Here's how the part is built. I have some questions about the finished solid (model axes, mm). Coordinates: 2 decimals unless noted, no trailing zeros.
from build123d import *

# Parameters (mm, degrees)
F0_W     = 97.8876724839
F0_H     = 45.6908610649
F1_DEPTH = 5


with BuildPart() as f1:
    # F0 (on Top) → F1 (new body)
    with BuildSketch(Plane.XY):
        with Locations((1.2231161818, -8.5958049167)):
            Rectangle(F0_W, F0_H)
        with BuildLine():
            Line((-26.666582018, -10.6564535441), (-26.666582018, -7.637935464))
            Line((-26.666582018, -7.637935464), (-19.8852024899, -7.637935464))
            Line((-19.8852024899, -7.637935464), (-19.8852024899, -16.4989879196))
            add(Edge.make_bspline(
                [(-19.8852024899, -16.4989879196), (-21.53472724, -17.0376082461), (-22.9897502054, -17.2545525443)],
                knots=[0, 0, 0, 1, 1, 1], degree=2))
            add(Edge.make_bspline(
                [(-22.9897502054, -17.2545525443), (-24.4447731709, -17.4714968425), (-25.9633832583, -17.4714968425)],
                knots=[0, 0, 0, 1, 1, 1], degree=2))
            add(Edge.make_bspline(
                [(-25.9633832583, -17.4714968425), (-29.8309764364, -17.4714968425), (-31.8713749652, -15.1973221304)],
                knots=[0, 0, 0, 1, 1, 1], degree=2))
            add(Edge.make_bspline(
                [(-31.8713749652, -15.1973221304), (-33.9117734939, -12.9231474183), (-33.9117734939, -8.666550671)],
                knots=[0, 0, 0, 1, 1, 1], degree=2))
            add(Edge.make_bspline(
                [(-33.9117734939, -8.666550671), (-33.9117734939, -4.5296473295), (-31.5440883084, -2.2161982186)],
                knots=[0, 0, 0, 1, 1, 1], degree=2))
            add(Edge.make_bspline(
                [(-31.5440883084, -2.2161982186), (-29.1764031229, 0.0972508923), (-24.9833934975, 0.0972508923)],
                knots=[0, 0, 0, 1, 1, 1], degree=2))
            add(Edge.make_bspline(
                [(-24.9833934975, 0.0972508923), (-22.3501385677, 0.0972508923), (-19.9076450035, -0.9538068283)],
                knots=[0, 0, 0, 1, 1, 1], degree=2))
            Line((-19.9076450035, -0.9538068283), (-21.1120599004, -3.8526315024))
            add(Edge.make_bspline(
                [(-21.1120599004, -3.8526315024), (-22.9822693676, -2.9175267688), (-25.0058360111, -2.9175267688)],
                knots=[0, 0, 0, 1, 1, 1], degree=2))
            add(Edge.make_bspline(
                [(-25.0058360111, -2.9175267688), (-27.3548191019, -2.9175267688), (-28.7686974591, -4.4959835591)],
                knots=[0, 0, 0, 1, 1, 1], degree=2))
            add(Edge.make_bspline(
                [(-28.7686974591, -4.4959835591), (-30.1825758163, -6.0744403494), (-30.1825758163, -8.7376186307)],
                knots=[0, 0, 0, 1, 1, 1], degree=2))
            add(Edge.make_bspline(
                [(-30.1825758163, -8.7376186307), (-30.1825758163, -11.5204903179), (-29.0436182508, -12.9867345402)],
                knots=[0, 0, 0, 1, 1, 1], degree=2))
            add(Edge.make_bspline(
                [(-29.0436182508, -12.9867345402), (-27.9046606852, -14.4529787625), (-25.7314772844, -14.4529787625)],
                knots=[0, 0, 0, 1, 1, 1], degree=2))
            add(Edge.make_bspline(
                [(-25.7314772844, -14.4529787625), (-24.5943899283, -14.4529787625), (-23.4273792208, -14.2210727885)],
                knots=[0, 0, 0, 1, 1, 1], degree=2))
            Line((-23.4273792208, -14.2210727885), (-23.4273792208, -10.6564535441))
            Line((-23.4273792208, -10.6564535441), (-26.666582018, -10.6564535441))
        make_face(mode=Mode.SUBTRACT)
        with BuildLine():
            add(Edge.make_bspline(
                [(-11.0559435953, -4.5951046609), (-10.0217177599, -3.9236994622), (-8.8060816063, -3.9236994622)],
                knots=[0, 0, 0, 1, 1, 1], degree=2))
            add(Edge.make_bspline(
                [(-8.8060816063, -3.9236994622), (-8.080440333, -3.9236994622), (-7.6016667094, -4.0284311923)],
                knots=[0, 0, 0, 1, 1, 1], degree=2))
            Line((-7.6016667094, -4.0284311923), (-7.8709768727, -7.3686253007))
            add(Edge.make_bspline(
                [(-7.8709768727, -7.3686253007), (-8.304865469, -7.2526723138), (-8.9220345932, -7.2526723138)],
                knots=[0, 0, 0, 1, 1, 1], degree=2))
            add(Edge.make_bspline(
                [(-8.9220345932, -7.2526723138), (-10.6276656273, -7.2526723138), (-11.5814724556, -8.1298005539)],
                knots=[0, 0, 0, 1, 1, 1], degree=2))
            add(Edge.make_bspline(
                [(-11.5814724556, -8.1298005539), (-12.5352792838, -9.006928794), (-12.5352792838, -10.5853855843)],
                knots=[0, 0, 0, 1, 1, 1], degree=2))
            Line((-12.5352792838, -10.5853855843), (-12.5352792838, -17.2358504497))
            Line((-12.5352792838, -17.2358504497), (-16.0998985283, -17.2358504497))
            Line((-16.0998985283, -17.2358504497), (-16.0998985283, -4.1668266929))
            Line((-16.0998985283, -4.1668266929), (-13.3993160577, -4.1668266929))
            Line((-13.3993160577, -4.1668266929), (-12.8719169879, -6.3661930263))
            Line((-12.8719169879, -6.3661930263), (-12.699857717, -6.3661930263))
            add(Edge.make_bspline(
                [(-12.699857717, -6.3661930263), (-12.0901694306, -5.2665098596), (-11.0559435953, -4.5951046609)],
                knots=[0, 0, 0, 1, 1, 1], degree=2))
        make_face(mode=Mode.SUBTRACT)
        with BuildLine():
            Line((5.5571271018, -17.2358504497), (3.0697485104, -17.2358504497))
            Line((3.0697485104, -17.2358504497), (2.3777710076, -15.4591514558))
            Line((2.3777710076, -15.4591514558), (2.2842605342, -15.4591514558))
            add(Edge.make_bspline(
                [(2.2842605342, -15.4591514558), (1.3865599899, -16.5924983929), (0.4327531617, -17.0319976177)],
                knots=[0, 0, 0, 1, 1, 1], degree=2))
            add(Edge.make_bspline(
                [(0.4327531617, -17.0319976177), (-0.5210536666, -17.4714968425), (-2.0508850108, -17.4714968425)],
                knots=[0, 0, 0, 1, 1, 1], degree=2))
            add(Edge.make_bspline(
                [(-2.0508850108, -17.4714968425), (-3.9323157348, -17.4714968425), (-5.0132968068, -16.3942561894)],
                knots=[0, 0, 0, 1, 1, 1], degree=2))
            add(Edge.make_bspline(
                [(-5.0132968068, -16.3942561894), (-6.0942778788, -15.3170155363), (-6.0942778788, -13.3308530822)],
                knots=[0, 0, 0, 1, 1, 1], degree=2))
            add(Edge.make_bspline(
                [(-6.0942778788, -13.3308530822), (-6.0942778788, -11.2511801546), (-4.6392549133, -10.263709556)],
                knots=[0, 0, 0, 1, 1, 1], degree=2))
            add(Edge.make_bspline(
                [(-4.6392549133, -10.263709556), (-3.1842319479, -9.2762389573), (-0.2517435033, -9.1715072271)],
                knots=[0, 0, 0, 1, 1, 1], degree=2))
            Line((-0.2517435033, -9.1715072271), (2.0186907899, -9.1004392674))
            Line((2.0186907899, -9.1004392674), (2.0186907899, -8.5281551704))
            add(Edge.make_bspline(
                [(2.0186907899, -8.5281551704), (2.0186907899, -6.5419927162), (-0.0160971104, -6.5419927162)],
                knots=[0, 0, 0, 1, 1, 1], degree=2))
            add(Edge.make_bspline(
                [(-0.0160971104, -6.5419927162), (-1.583332644, -6.5419927162), (-3.7004097608, -7.4883187066)],
                knots=[0, 0, 0, 1, 1, 1], degree=2))
            Line((-3.7004097608, -7.4883187066), (-4.8786417252, -5.0794889129))
            add(Edge.make_bspline(
                [(-4.8786417252, -5.0794889129), (-2.6231691077, -3.8975165296), (0.1222983901, -3.8975165296)],
                knots=[0, 0, 0, 1, 1, 1], degree=2))
            add(Edge.make_bspline(
                [(0.1222983901, -3.8975165296), (2.751812901, -3.8975165296), (4.1544700014, -5.043954933)],
                knots=[0, 0, 0, 1, 1, 1], degree=2))
            add(Edge.make_bspline(
                [(4.1544700014, -5.043954933), (5.5571271018, -6.1903933364), (5.5571271018, -8.5281551704)],
                knots=[0, 0, 0, 1, 1, 1], degree=2))
            Line((5.5571271018, -8.5281551704), (5.5571271018, -17.2358504497))
        make_face(mode=Mode.SUBTRACT)
        with BuildLine():
            add(Edge.make_bspline(
                [(16.7634222292, -17.2601631727), (15.8806833607, -17.4714968425), (14.5378729632, -17.4714968425)],
                knots=[0, 0, 0, 1, 1, 1], degree=2))
            add(Edge.make_bspline(
                [(14.5378729632, -17.4714968425), (8.4372496813, -17.4714968425), (8.4372496813, -10.772406531)],
                knots=[0, 0, 0, 1, 1, 1], degree=2))
            add(Edge.make_bspline(
                [(8.4372496813, -10.772406531), (8.4372496813, -7.4396932605), (10.0961254787, -5.6816963613)],
                knots=[0, 0, 0, 1, 1, 1], degree=2))
            add(Edge.make_bspline(
                [(10.0961254787, -5.6816963613), (11.7550012761, -3.9236994622), (14.8520681537, -3.9236994622)],
                knots=[0, 0, 0, 1, 1, 1], degree=2))
            add(Edge.make_bspline(
                [(14.8520681537, -3.9236994622), (17.118762028, -3.9236994622), (18.9216439544, -4.8101787496)],
                knots=[0, 0, 0, 1, 1, 1], degree=2))
            Line((18.9216439544, -4.8101787496), (17.8668458149, -7.5706079232))
            add(Edge.make_bspline(
                [(17.8668458149, -7.5706079232), (17.0252515546, -7.2302298002), (16.3014804908, -7.013285502)],
                knots=[0, 0, 0, 1, 1, 1], degree=2))
            add(Edge.make_bspline(
                [(16.3014804908, -7.013285502), (15.577709427, -6.7963412038), (14.8520681537, -6.7963412038)],
                knots=[0, 0, 0, 1, 1, 1], degree=2))
            add(Edge.make_bspline(
                [(14.8520681537, -6.7963412038), (12.0691964666, -6.7963412038), (12.0691964666, -10.7499640174)],
                knots=[0, 0, 0, 1, 1, 1], degree=2))
            add(Edge.make_bspline(
                [(12.0691964666, -10.7499640174), (12.0691964666, -14.5838934252), (14.8520681537, -14.5838934252)],
                knots=[0, 0, 0, 1, 1, 1], degree=2))
            add(Edge.make_bspline(
                [(14.8520681537, -14.5838934252), (15.8806833607, -14.5838934252), (16.7578116008, -14.3089726335)],
                knots=[0, 0, 0, 1, 1, 1], degree=2))
            add(Edge.make_bspline(
                [(16.7578116008, -14.3089726335), (17.6349398409, -14.0340518418), (18.5101978716, -13.4468060691)],
                knots=[0, 0, 0, 1, 1, 1], degree=2))
            Line((18.5101978716, -13.4468060691), (18.5101978716, -16.4989879196))
            add(Edge.make_bspline(
                [(18.5101978716, -16.4989879196), (17.6461610977, -17.0488295029), (16.7634222292, -17.2601631727)],
                knots=[0, 0, 0, 1, 1, 1], degree=2))
        make_face(mode=Mode.SUBTRACT)
        with BuildLine():
            add(Edge.make_bspline(
                [(30.0493902842, -17.2433312875), (28.9871113068, -17.4714968425), (27.4535395437, -17.4714968425)],
                knots=[0, 0, 0, 1, 1, 1], degree=2))
            add(Edge.make_bspline(
                [(27.4535395437, -17.4714968425), (24.300366382, -17.4714968425), (22.5236673882, -15.7284616191)],
                knots=[0, 0, 0, 1, 1, 1], degree=2))
            add(Edge.make_bspline(
                [(22.5236673882, -15.7284616191), (20.7469683943, -13.9854263957), (20.7469683943, -10.7948490446)],
                knots=[0, 0, 0, 1, 1, 1], degree=2))
            add(Edge.make_bspline(
                [(20.7469683943, -10.7948490446), (20.7469683943, -7.5107612202), (22.3890123065, -5.7172303412)],
                knots=[0, 0, 0, 1, 1, 1], degree=2))
            add(Edge.make_bspline(
                [(22.3890123065, -5.7172303412), (24.0310562187, -3.9236994622), (26.9298808929, -3.9236994622)],
                knots=[0, 0, 0, 1, 1, 1], degree=2))
            add(Edge.make_bspline(
                [(26.9298808929, -3.9236994622), (29.6977909043, -3.9236994622), (31.2407137148, -5.500286043)],
                knots=[0, 0, 0, 1, 1, 1], degree=2))
            add(Edge.make_bspline(
                [(31.2407137148, -5.500286043), (32.7836365252, -7.0768726239), (32.7836365252, -9.859744311)],
                knots=[0, 0, 0, 1, 1, 1], degree=2))
            Line((32.7836365252, -9.859744311), (32.7836365252, -11.5915582777))
            Line((32.7836365252, -11.5915582777), (24.356472666, -11.5915582777))
            add(Edge.make_bspline(
                [(24.356472666, -11.5915582777), (24.416319369, -13.110168365), (25.2579136292, -13.9629838821)],
                knots=[0, 0, 0, 1, 1, 1], degree=2))
            add(Edge.make_bspline(
                [(25.2579136292, -13.9629838821), (26.0995078894, -14.8157993991), (27.6181179768, -14.8157993991)],
                knots=[0, 0, 0, 1, 1, 1], degree=2))
            add(Edge.make_bspline(
                [(27.6181179768, -14.8157993991), (28.8000903601, -14.8157993991), (29.8511480806, -14.5708019589)],
                knots=[0, 0, 0, 1, 1, 1], degree=2))
            add(Edge.make_bspline(
                [(29.8511480806, -14.5708019589), (30.9022058012, -14.3258045187), (32.0467739951, -13.7871841921)],
                knots=[0, 0, 0, 1, 1, 1], degree=2))
            Line((32.0467739951, -13.7871841921), (32.0467739951, -16.5476133657))
            add(Edge.make_bspline(
                [(32.0467739951, -16.5476133657), (31.1116692615, -17.0151657325), (30.0493902842, -17.2433312875)],
                knots=[0, 0, 0, 1, 1, 1], degree=2))
        make_face(mode=Mode.SUBTRACT)
    extrude(amount=F1_DEPTH)


solid = f1.part
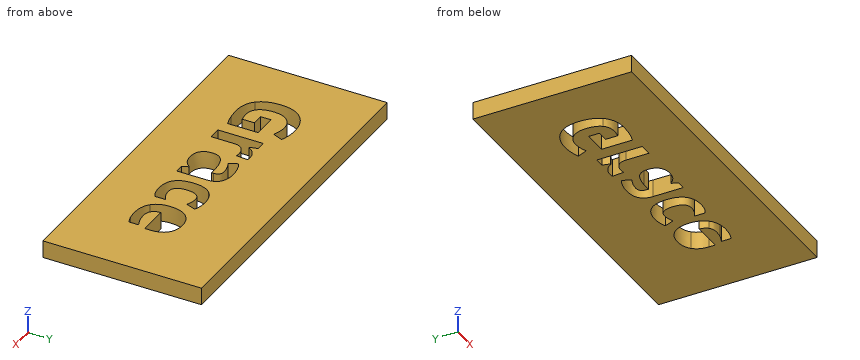
Q1. Suppose I cut it at A-A on z = 3.65. State how many separate pieces and enclosed holes the cut face has, and give its area (3 significant figures).
Q2. Please list where these lines run through material, in increasing order: probe 1 along Y at (x, z) = (14.5, 1.8); probe 2 along X at (y, z) = (-15, 2.6); probe 3 along Y at (x, z) = (1, 4.6).
Q3. Will this pin go through, and if not, where does the flat tip stop? P1, Ø2, axis at x = 8, y = -21.5, coming from the -Z side.
Check values:
1. separate pieces: 1
1. enclosed holes: 5
1. area: 3,960 mm2
2. probe 1: y = -31.44 to -17.47, -14.57 to -6.81, -3.93 to 14.25
2. probe 2: x = -47.72 to -32.04, -19.89 to -16.1, -12.54 to -5.85, 5.56 to 9.38, 18.51 to 21.9, 32.05 to 50.17
2. probe 3: y = -31.44 to -16.71, -9.13 to -6.71, -3.93 to 14.25
3. P1: stops at z = 0
